```python
from build123d import *

# Parameters (mm, degrees)
ESQUISSE1_W                  = 62
ESQUISSE1_H                  = 60
BOSS_EXTRU_1_DEPTH           = 10
ESQUISSE3_R                  = 5
BOSS_EXTRU_2_DEPTH           = 5
ESQUISSE4_R                  = 3.5
BOSS_EXTRU_3_DEPTH           = 2
ESQUISSE5_R                  = 1.625
ENL_V_MAT_EXTRU_2_DEPTH      = 88.93747779
BOSS_EXTRU_4_DEPTH           = 3
ESQUISSE9_R                  = 11
ESQUISSE9_R_2                = 1.625
ESQUISSE9_R_3                = 1.5
ENL_V_MAT_EXTRU_4_DEPTH      = 10
BOSS_EXTRU_6_DEPTH           = 63
ENL_V_MAT_EXTRU_6_DEPTH      = 4
ENL_V_MAT_EXTRU_7_DEPTH      = 102
ENL_V_MAT_EXTRU_8_DEPTH      = 23
ENL_V_MAT_EXTRU_8_DEPTH_BACK = 1
ESQUISSE19_W                 = 42
ESQUISSE19_H                 = 42
CHANFREIN1_SIZE              = 1
CONG_1_R                     = 10
ESQUISSE20_W                 = 96.792413771
ESQUISSE20_H                 = 78.280203487
ENL_V_MAT_EXTRU_10_DEPTH     = 107.575890285


with BuildPart() as part:
    # Esquisse1 → Boss.-Extru.1 (new body)
    with BuildSketch(Plane.XY):
        with Locations((31, 30)):
            Rectangle(ESQUISSE1_W, ESQUISSE1_H)
    extrude(amount=BOSS_EXTRU_1_DEPTH)

    # Esquisse3 → Boss.-Extru.2 (add)
    with BuildSketch(Plane.XY.offset(10)):
        with Locations(Location((6, 52.5, 0), (0, 0, 180))):
            Circle(ESQUISSE3_R)
        with Locations(Location((56, 7.5, 0), (0, 0, 180))):
            Circle(ESQUISSE3_R)
        with Locations(Location((6, 7.5, 0), (0, 0, 180))):
            Circle(ESQUISSE3_R)
        with Locations(Location((56, 52.5, 0), (0, 0, 180))):
            Circle(ESQUISSE3_R)
    extrude(amount=BOSS_EXTRU_2_DEPTH)

    # Esquisse4 → Boss.-Extru.3 (add)
    with BuildSketch(Plane.XY.offset(15)):
        with Locations((6, 52.5)):
            Circle(ESQUISSE4_R)
        with Locations((56, 52.5)):
            Circle(ESQUISSE4_R)
        with Locations((56, 7.5)):
            Circle(ESQUISSE4_R)
        with Locations((6, 7.5)):
            Circle(ESQUISSE4_R)
    extrude(amount=BOSS_EXTRU_3_DEPTH)

    # Esquisse5 → Enlèv. mat.-Extru.2 (cut, through all)
    with BuildSketch(Plane.XY.offset(17)):
        with Locations((6, 52.5)):
            Circle(ESQUISSE5_R)
        with Locations((56, 52.5)):
            Circle(ESQUISSE5_R)
        with Locations((56, 7.5)):
            Circle(ESQUISSE5_R)
        with Locations((6, 7.5)):
            Circle(ESQUISSE5_R)
    extrude(amount=-ENL_V_MAT_EXTRU_2_DEPTH, mode=Mode.SUBTRACT)

    # Esquisse7 → Boss.-Extru.4 (add, symmetric)
    with BuildSketch(Plane(origin=(0, 60, 0), x_dir=(1, 0, 0), z_dir=(0, 1, 0))):
        with BuildLine():
            Line((0, 0), (0, -10))
            Line((0, -10), (62, -10))
            Line((62, -10), (62, 0))
            ThreePointArc((62, 0), (61.543258885, 25.799206928), (56, 51))
            Line((56, 51), (6, 51))
            ThreePointArc((6, 51), (0.456741115, 25.799206928), (0, 0))
        make_face()
    extrude(amount=BOSS_EXTRU_4_DEPTH, both=True)

    # Esquisse9 → Enlèv. mat.-Extru.4 (cut)
    with BuildSketch(Plane(origin=(0, 63, 0), x_dir=(1, 0, 0), z_dir=(0, 1, 0))):
        with Locations(Location((31, 30, 0), (0, 0, 270))):
            Circle(ESQUISSE9_R)
        with Locations(Location((46.5, 14.5, 0), (0, 0, 270))):
            Circle(ESQUISSE9_R_2)
        with Locations(Location((15.5, 14.5, 0), (0, 0, 270))):
            Circle(ESQUISSE9_R_2)
        with Locations(Location((15.5, 45.5, 0), (0, 0, 270))):
            Circle(ESQUISSE9_R_2)
        with Locations(Location((46.5, 45.5, 0), (0, 0, 270))):
            Circle(ESQUISSE9_R_2)
        with Locations(Location((56, 18, 0), (0, 0, 270))):
            Circle(ESQUISSE9_R_3)
        with Locations(Location((6, 18, 0), (0, 0, 270))):
            Circle(ESQUISSE9_R_3)
    extrude(amount=-ENL_V_MAT_EXTRU_4_DEPTH, mode=Mode.SUBTRACT)

    # Esquisse14 → Boss.-Extru.6 (add)
    with BuildSketch(Plane(origin=(0, 63, 0), x_dir=(1, 0, 0), z_dir=(0, 1, 0))):
        with BuildLine():
            Line((0, 0), (0, -10))
            Line((0, -10), (-6.92820323, -6))
            ThreePointArc((-6.92820323, -6), (-4.721429116, 23.465606932), (6, 51))
            Line((6, 51), (11.044473074, 51))
            ThreePointArc((11.044473074, 51), (2.937001082, 26.059854184), (0, 0))
        make_face()
    boss_extru_6 = extrude(amount=-BOSS_EXTRU_6_DEPTH)

    # Symétrie1: Boss.-Extru.6 across plane
    add(boss_extru_6.mirror(Plane(origin=(31, 0, 0), x_dir=(0, 0, 1), z_dir=(1, 0, 0))))

    # Esquisse16 → Enlèv. mat.-Extru.6 (cut)
    with BuildSketch(Plane.XZ.offset(-57)):
        Polygon((10.041451884, -18), (8.020725942, -14.5), (3.979274058, -14.5), (1.958548116, -18), (3.979274058, -21.5), (8.020725942, -21.5), align=None)
        Polygon((60.041451884, -18), (58.020725942, -14.5), (53.979274058, -14.5), (51.958548116, -18), (53.979274058, -21.5), (58.020725942, -21.5), align=None)
    extrude(amount=-ENL_V_MAT_EXTRU_6_DEPTH, mode=Mode.SUBTRACT)

    # Esquisse18 → Enlèv. mat.-Extru.7 (cut, symmetric)
    with BuildSketch(Plane(origin=(0, 0, 0), x_dir=(0, 0, -1), z_dir=(1, 0, 0))):
        with BuildLine():
            Line((51, 53), (51, 0))
            Line((51, 0), (0, 0))
            ThreePointArc((0, 0), (17.977874458, 33.738271748), (51, 53))
        make_face()
    extrude(amount=ENL_V_MAT_EXTRU_7_DEPTH, both=True, mode=Mode.SUBTRACT)

    # Esquisse19 → Enlèv. mat.-Extru.8 (cut, two sides: drawn at the far end of the back side and taken through both)
    with BuildSketch(Plane.XZ.offset(-57).offset(-ENL_V_MAT_EXTRU_8_DEPTH_BACK)):
        with Locations((31, -30)):
            Rectangle(ESQUISSE19_W, ESQUISSE19_H)
    extrude(amount=ENL_V_MAT_EXTRU_8_DEPTH + ENL_V_MAT_EXTRU_8_DEPTH_BACK, mode=Mode.SUBTRACT)

    # Chanfrein1
    chanfrein1_edges = [part.edges().sort_by_distance(p)[0] for p in [
        (31, 63, -41),
    ]]
    chamfer(chanfrein1_edges, length=CHANFREIN1_SIZE)

    # Congé1
    cong_1_edges = [part.edges().sort_by_distance(p)[0] for p in [
        (-6.92820323, 31.5, 6),
        (68.92820323, 31.5, 6),
    ]]
    fillet(cong_1_edges, radius=CONG_1_R)

    # Esquisse20 → Enlèv. mat.-Extru.10 (cut, through all)
    with BuildSketch(Plane(origin=(0, 63, 0), x_dir=(1, 0, 0), z_dir=(0, 1, 0))):
        with Locations((33.820908233, 33.83729602)):
            Rectangle(ESQUISSE20_W, ESQUISSE20_H)
    extrude(amount=-ENL_V_MAT_EXTRU_10_DEPTH, mode=Mode.SUBTRACT)


solid = part.part
```
Check sheet for the modelled part. Datum: model origin and axes. Units: mm. A direction names the side the tool comes from. Coordinates: 2 decimals unless noted, no trailing zeros. Order: outer loops, then holes, each group sorted by start corner. A loop starts at its lowest first (then second) coordinate and runs counter-clockwise, first axis right, second up. Notation, with made-up numbers: M 5.5,-30.5 L 9.5,-30.5 A10 cw 9.5,-18.5 Z; hole C 42.25,-33.5 d5. An arc over 180 degrees is marked long. One line per question, with ' | ' between items. Start each with the question number.
Item 1: Access from +Z, -Z, +X, -X, +Y, -Y to the whole of each face (thin tool, end or side, straight path). Record for faces 1 (the cylindrical face through (5.648, 50.914, 11.233)), 2 (the cylindrical face through (59.685, 4.121, 12.465)).
Item 2: Sectioned sample at D-D on z = 6.5. Record the cut outline in (x, y) (3 decimals).
Item 3: Sectioned sample at C-C on y = 7.5. Count the separate pieces of the cut face and the enclosed holes in it, and give its area (3 significant figures).
Item 4: Mould release check, pull along Y, two halves, no side actions. Record for faces 3 (the flat face through (54, 11, 15)), 4 (the flat face through (30, 0, 8)), 5 (the cylindrical face through (66.14, 31.059, 7.265)): pulls with the +Y half, pulls with the -Y half, needs draft (parallel to the pull), parting line crosses it, or undercut.
Item 5: Sectioned sample at A-A on z = 11. Record the cut outline in (x, y) (3 decimals), and give its area (3 significant figures).
Item 6: Gauge pin test, flat ends, axial feed: P1, Ø6, axis at y = 44.5, z = 9, coming from the +X side; P2, Ø5, axis at x = 15.5, y = 21.5, coming from the +Z side; P3, Ø6, axis at y = 34, z = 7, coming from the -X side. Record the tip position at first contact, or that the pin passes through.
Item 7: Material ranges on line 1 (Y direction, x = 56, z = 8.5) (3 decimals); line 2 (Y direction, x = 56, z = 10.5) (3 decimals); line 3 (Z direction, x = 17, y = 41.5), recorded low to high.
Item 8: Sectioned sample at B-B on x = 56. Record the cut outline in (y, z) (3 decimals).
Answer below:
1) face 1: +Z, -Z | face 2: +Z
2) outline: M -4.852,0 L 66.852,0 L 66.852,63 L -4.852,63 Z; hole C 6,7.5 d3.25; hole C 6,52.5 d3.25; hole C 56,7.5 d3.25; hole C 56,52.5 d3.25
3) separate pieces: 3 | enclosed holes: 0 | area: 375 mm^2
4) face 3: undercut | face 4: pulls with the -Y half | face 5: needs draft
5) outline: C 6,7.5 d10; C 6,52.5 d10; C 56,7.5 d10; C 56,52.5 d10; hole C 6,7.5 d3.25; hole C 6,52.5 d3.25; hole C 56,7.5 d3.25; hole C 56,52.5 d3.25 | area: 281 mm^2
6) P1: stops at x = 67.24 | P2: stops at z = 10 | P3: stops at x = -5.71
7) line 1: y = 0 to 5.875, 9.125 to 50.875, 54.125 to 63 | line 2: y = 2.5 to 5.875, 9.125 to 12.5, 47.5 to 50.875, 54.125 to 57.5 | line 3: z = 5.3 to 10
8) outline: M 0,5.303 L 5.875,5.303 L 5.875,17 L 4,17 L 4,15 L 2.5,15 L 2.5,10 L 0,10 Z; M 9.125,5.303 L 50.875,5.303 L 50.875,17 L 49,17 L 49,15 L 47.5,15 L 47.5,10 L 12.5,10 L 12.5,15 L 11,15 L 11,17 L 9.125,17 Z; M 54.125,5.303 L 63,5.303 L 63,10 L 57.5,10 L 57.5,15 L 56,15 L 56,17 L 54.125,17 Z
